Verification items for the finished model (mm, model axes). Face numbers are marked on the shaded views. A direction names the side the tool comes from. Coordinates: 2 decimals unless noted, no trailing zeros. Write each loop counter-clockwise with the first axis right and the second up, starting at its lowest first coordinate (ties: lowest second). Pieces come first, ordered by that corner, then holes. Notation, with made-up numbers: (20, -6.5) -> (52, -6.5) arc R16 ccw to (52, 4.5) -> close; hole circle Ø11 at (4, 74.25). An arc over 180 degrees is marked (long way). Write item = value, one per line. Start each with the question number.
(1) Section check B-B (z = 46.5). Record the cut outline in (x, y), plus the area to 3 significant figures.
(2) Section check C-C (x = 35). Record the cut outline in (y, z).
(3) Material ranges on probe 1 along Y at (x, z) = (-15.24, 4.25); probe 2 along Z at (x, y) = (36, 0); probe 3 along X at (y, z) = (6.5, 28.5), recorded low to high. Write a range as [from, to].
(4) Section check A-A (z = 31.75). Record the cut outline in (x, y), plus the area to 3 significant figures.
(5) Section check D-D (y = 0). Record the cut outline in (x, z).
(6) Mould release check, pull along Z, two halves, no side actions. Record for the marked faces 3, 4 and 5: released by +Z, released by -Z, zero draft, split by the parting line, or undercut.
(7) Gauge pin test, flat end, axial feed: pin 1 Ø1.5 at (x, y) = (-4, 24) entering from +Z. Record the tip position at first contact, or that the pin passes through.
(8) Set-up check for the marked faces 1 and 2: record each of +Z, -Z, +X, -X, +Y, -Y from which the full face is reachable in a straight line by a thin tool's end or side.
```python
from build123d import *

# Parameters (mm, degrees)
F0_W     = 101.6
F0_H     = 76.2
F1_DEPTH = 50.8
F2_W     = 50.8
F2_H     = 76.2
F3_DEPTH = 38.1
F4_SIZE  = 25.4
F5_R     = 6.35
F6_DEPTH = 101.601
F7_R     = 6.35
F8_DEPTH = 12.7


with BuildPart() as f1:
    # F0 (on Top) → F1 (new body)
    with BuildSketch(Plane.XY):
        Rectangle(F0_W, F0_H)
    extrude(amount=F1_DEPTH)

    # F2 (on face) → F3 (cut)
    with BuildSketch(Plane.XY.offset(50.8)):
        Rectangle(F2_W, F2_H)
    extrude(amount=-F3_DEPTH, mode=Mode.SUBTRACT)

    # F4
    f4_edges = [f1.edges().sort_by_distance(p)[0] for p in [
        (-38.1, -38.1, 50.8),
        (38.1, -38.1, 50.8),
        (-38.1, 38.1, 50.8),
        (38.1, 38.1, 50.8),
    ]]
    chamfer(f4_edges, length=F4_SIZE)

    # F5 (on face) → F6 (cut, through all)
    with BuildSketch(Plane.YZ.offset(50.8)):
        with Locations((0, 31.75)):
            Circle(F5_R)
    extrude(amount=-F6_DEPTH, mode=Mode.SUBTRACT)

    # F7 (on face) → F8 (cut, through all)
    with BuildSketch(Plane.XY.offset(12.7)):
        with Locations((-15.24, -25.4)):
            Circle(F7_R)
        with Locations((-15.24, 25.4)):
            Circle(F7_R)
        with Locations((15.24, -25.4)):
            Circle(F7_R)
        with Locations((15.24, 25.4)):
            Circle(F7_R)
    extrude(amount=-F8_DEPTH, mode=Mode.SUBTRACT)


solid = f1.part
```
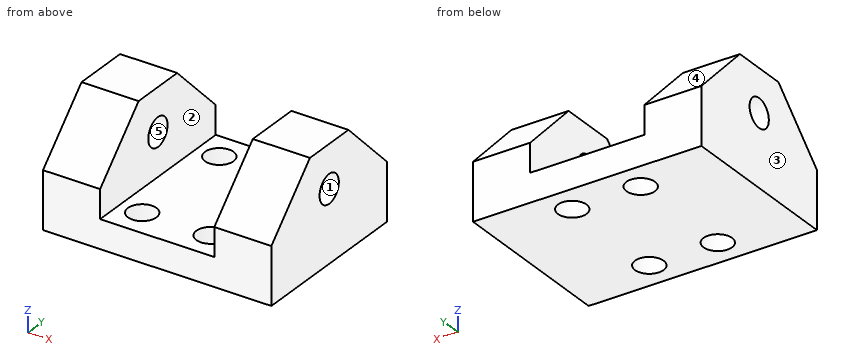
Response:
q1.outline = (-50.8, -17) -> (-25.4, -17) -> (-25.4, 17) -> (-50.8, 17) -> close; (25.4, -17) -> (50.8, -17) -> (50.8, 17) -> (25.4, 17) -> close
q1.area = 1,730 mm2
q2.outline = (-38.1, 0) -> (38.1, 0) -> (38.1, 25.4) -> (12.7, 50.8) -> (-12.7, 50.8) -> (-38.1, 25.4) -> close; hole circle Ø12.7 at (0, 31.75)
q3.probe_1 = [-38.1, -31.75], [-19.05, 19.05], [31.75, 38.1]
q3.probe_2 = [0, 25.4], [38.1, 50.8]
q3.probe_3 = [-50.8, -25.4], [25.4, 50.8]
q4.outline = (-50.8, -31.75) -> (-25.4, -31.75) -> (-25.4, -6.35) -> (-50.8, -6.35) -> close; (-50.8, 6.35) -> (-25.4, 6.35) -> (-25.4, 31.75) -> (-50.8, 31.75) -> close; (25.4, -31.75) -> (50.8, -31.75) -> (50.8, -6.35) -> (25.4, -6.35) -> close; (25.4, 6.35) -> (50.8, 6.35) -> (50.8, 31.75) -> (25.4, 31.75) -> close
q4.area = 2,580 mm2
q5.outline = (-50.8, 0) -> (50.8, 0) -> (50.8, 25.4) -> (25.4, 25.4) -> (25.4, 12.7) -> (-25.4, 12.7) -> (-25.4, 25.4) -> (-50.8, 25.4) -> close; (-50.8, 38.1) -> (-25.4, 38.1) -> (-25.4, 50.8) -> (-50.8, 50.8) -> close; (25.4, 38.1) -> (50.8, 38.1) -> (50.8, 50.8) -> (25.4, 50.8) -> close
q6.face_3 = zero draft
q6.face_4 = released by +Z
q6.face_5 = undercut
q7.pin_1 = 12.7
q8.face_1 = +X, -X
q8.face_2 = +Z, +Y, -Y
